CAD build for the part. Positions are in the model's coordinates, mm. A direction names the side the tool comes from. Round coordinates to 2 decimals unless told otherwise and drop trailing zeros. Write each loop counter-clockwise with the first axis right and the second up, starting at its lowest first coordinate (ties: lowest second). Pieces come first, ordered by that corner, then holes. Notation, with made-up numbers: (86.25, -23.75) - (111.25, -23.75) arc R33 ccw to (111.25, 15.25) - close; hole circle Ø1 at (-9, -23.5). An arc over 180 degrees is marked (long way). Use one line per item in the form item = value. Start each with the question number.
Item 1: Pull direction X, two halves, no side cores. Call faces 1 (the flat face through (57.074, 23, 7)), 2 (the flat face through (53, 2, -9.576)), 3 (the cylindrical face through (51.904, 4.037, -5.193)): +X half, -X half, draft (parallel to the pull), parting line (faces both ways), or undercut.
Item 2: Band-saw the part on C-C, the plane y = 40. List the corners of the cut face in (x, z), and give its area (3 significant figures).
Item 3: Band-saw the part on A-A, the plane z = -1.75. List the corners of the cut face in (x, y), and give its area (3 significant figures).
Item 4: Drill centre lines: L1, parallel to Z at x = 30, y = 40; L2, parallel to X at y = 39, z = -1; L3, parallel to Y at x = 51, z = -8. Where is each one in solid material? Low to high.
Item 5: Band-saw the part on B-B, the plane x = 6. List the corners of the cut face in (y, z), and give its area (3 significant figures).
Item 6: Pin check, flat tips, straight feed: pin 1 (3 mm diameter, centred on x = 3.5, y = 42.5, fed in from -Z); pin 2 (0.8 mm diameter, centred on x = 52.5, y = 42.5, fed in from -Z); pin 3 (2 mm diameter, centred on x = 49, y = 8, fed in from -Z). Stop position of each tip, or through.
Item 7: Tool access for faces 4 (the flat face through (4, 42, -0.686)), 5 (the flat face through (28, 0, 7)): list every direction of +Z, -Z, +X, -X, +Y, -Y with a clear straight run to the whole face (end or side of a thin tool).
Item 8: Band-saw the part on D-D, the plane x = 53.5. List the corners of the cut face in (y, z), and give its area (3 significant figures).
from build123d import *

# Parameters (mm, degrees)
SKETCH1_W           = 57.0738
SKETCH1_H           = 45.6438
BOSS_EXTRUDE1_DEPTH = 14.8082
SKETCH2_R           = 3.5687
BOSS_EXTRUDE2_DEPTH = 9.5758
SKETCH3_R           = 1.3462
CUT_EXTRUDE1_DEPTH  = 8.89


with BuildPart() as part:
    # Sketch1 → Boss-Extrude1 (new body)
    with BuildSketch(Plane.XY):
        with Locations((28.5369, 22.8219)):
            Rectangle(SKETCH1_W, SKETCH1_H)
    extrude(amount=BOSS_EXTRUDE1_DEPTH)

    # Sketch2 → Boss-Extrude2 (add)
    with BuildSketch(Plane(origin=(0, 0, 0), x_dir=(-1, 0, 0), z_dir=(0, 0, -1))):
        with Locations((-3.8862, 42.0116)):
            Circle(SKETCH2_R)
        with Locations((-3.8862, 3.6322)):
            Circle(SKETCH2_R)
        with Locations((-53.1876, 3.6322)):
            Circle(SKETCH2_R)
        with Locations((-53.1876, 42.0116)):
            Circle(SKETCH2_R)
    extrude(amount=BOSS_EXTRUDE2_DEPTH)

    # Sketch3 → Cut-Extrude1 (cut)
    with BuildSketch(Plane(origin=(0, 0, -9.5758), x_dir=(-1, 0, 0), z_dir=(0, 0, -1))):
        with Locations((-3.8862, 3.6322)):
            Circle(SKETCH3_R)
        with Locations((-53.1876, 3.6322)):
            Circle(SKETCH3_R)
        with Locations((-53.1876, 42.0116)):
            Circle(SKETCH3_R)
        with Locations((-3.8862, 42.0116)):
            Circle(SKETCH3_R)
    extrude(amount=-CUT_EXTRUDE1_DEPTH, mode=Mode.SUBTRACT)


solid = part.part
Determined:
q1.face_1 = +X half
q1.face_2 = draft
q1.face_3 = undercut
q2.outline = (0, 0) - (0.94, 0) - (0.94, -9.58) - (6.83, -9.58) - (6.83, 0) - (50.24, 0) - (50.24, -9.58) - (56.14, -9.58) - (56.14, 0) - (57.07, 0) - (57.07, 14.81) - (0, 14.81) - close
q2.area = 958 mm²
q3.outline = circle Ø7.14 at (3.89, 3.63); circle Ø7.14 at (3.89, 42.01); circle Ø7.14 at (53.19, 3.63); circle Ø7.14 at (53.19, 42.01); hole circle Ø2.69 at (3.89, 3.63); hole circle Ø2.69 at (3.89, 42.01); hole circle Ø2.69 at (53.19, 3.63); hole circle Ø2.69 at (53.19, 42.01)
q3.area = 137 mm²
q4.L1 = 0 to 14.81
q4.L2 = 1.97 to 5.8, 51.27 to 55.1
q4.L3 = 0.81 to 6.45, 39.19 to 44.83
q5.outline = (0, 0) - (0.76, 0) - (0.76, -9.58) - (6.51, -9.58) - (6.51, 0) - (39.14, 0) - (39.14, -9.58) - (44.89, -9.58) - (44.89, 0) - (45.64, 0) - (45.64, 14.81) - (0, 14.81) - close
q5.area = 786 mm²
q6.pin_1 = -9.58
q6.pin_2 = -0.69
q6.pin_3 = 0
q7.face_4 = -Z
q7.face_5 = +Z, -Z, +X, -X, -Y
q8.outline = (0, 0) - (0.08, 0) - (0.08, -9.58) - (2.32, -9.58) - (2.32, -0.69) - (4.94, -0.69) - (4.94, -9.58) - (7.19, -9.58) - (7.19, 0) - (38.46, 0) - (38.46, -9.58) - (40.7, -9.58) - (40.7, -0.69) - (43.32, -0.69) - (43.32, -9.58) - (45.57, -9.58) - (45.57, 0) - (45.64, 0) - (45.64, 14.81) - (0, 14.81) - close
q8.area = 766 mm²
